```python
from build123d import *

# Parameters (mm, degrees)
F0_W          = 38.1
F0_H          = 6.35
F0_R          = 1.5875
F1_DEPTH      = 3.175
F1_DEPTH_BACK = 3.175


with BuildPart() as f1:
    # F0 (on Right) → F1 (new body, two sides)
    with BuildSketch(Plane.YZ) as f1_sk:
        Rectangle(F0_W, F0_H)
        with Locations((-12.7, 0)):
            Circle(F0_R, mode=Mode.SUBTRACT)
        with Locations((-6.35, 0)):
            Circle(F0_R, mode=Mode.SUBTRACT)
        Circle(F0_R, mode=Mode.SUBTRACT)
        with Locations((6.35, 0)):
            Circle(F0_R, mode=Mode.SUBTRACT)
        with Locations((12.7, 0)):
            Circle(F0_R, mode=Mode.SUBTRACT)
    extrude(amount=F1_DEPTH)
    extrude(f1_sk.sketch, amount=-F1_DEPTH_BACK)


solid = f1.part
```
Work out the finished part from the listing and answer in its coordinate system (mm). Give positions to 0.01 mm unless a question says otherwise; leave off trailing zeros. Loops run counter-clockwise (first coordinate to the right, second up) from the corner with the lowest first, then second, coordinate; pieces in that order, holes last. Notation, with made-up numbers: (-31.75, 71) -> (5.25, 71) arc R22 ccw to (5.25, 107) -> close; hole circle Ø8 at (25, -15.75). An arc over 180 degrees is marked (long way). Put each result on its own line as item: value. Start each with the question number.
Item 1: The mould has two halves that part along Z. Classify faces 1 (the face through (0, 0, -3.175)), 2 (the face through (-0.04, -0.34, -1.55)), 3 (the face through (0, -19.05, 0)): released by +Z, released by -Z, zero draft, split by the parting line, or undercut.
Item 2: The part is cut by section A-A (y = 0). Give the vertices of the cut face in (x, z) (1 decimal).
Item 3: The part is cut by section B-B (x = 2). State how many separate pieces and enclosed holes the cut face has, then the cut area to 3 significant figures.
Item 4: The part is cut by section D-D (y = 12.5). Give the vertices of the cut face in (x, z) (3 decimals).
Item 5: Find the intervals of material crossed by L1, parallel to Z at x = 0.5, y = -6.35 (1 decimal); L2, parallel to Y at x = 0, z = 0.5; L3, parallel to Y at x = 1.5, z = 0.25, in increasing order. Write a range as [from, to].
Item 6: This flat-tipped pin is pushed along its axis until it touches: P1, Ø1.9, axis at y = -6.35, z = 0, coming from the -X side. Where does it stop, or does it pass through?
Answers below:
1. face 1: released by -Z
1. face 2: undercut
1. face 3: zero draft
2. outline: (-3.2, -3.2) -> (3.2, -3.2) -> (3.2, -1.6) -> (-3.2, -1.6) -> close; (-3.2, 1.6) -> (3.2, 1.6) -> (3.2, 3.2) -> (-3.2, 3.2) -> close
3. separate pieces: 1
3. enclosed holes: 5
3. area: 202 mm2
4. outline: (-3.175, -3.175) -> (3.175, -3.175) -> (3.175, -1.575) -> (-3.175, -1.575) -> close; (-3.175, 1.575) -> (3.175, 1.575) -> (3.175, 3.175) -> (-3.175, 3.175) -> close
5. L1: [-3.2, -1.6], [1.6, 3.2]
5. L2: [-19.05, -14.21], [-11.19, -7.86], [-4.84, -1.51], [1.51, 4.84], [7.86, 11.19], [14.21, 19.05]
5. L3: [-19.05, -14.27], [-11.13, -7.92], [-4.78, -1.57], [1.57, 4.78], [7.92, 11.13], [14.27, 19.05]
6. P1: through
